The listing builds one solid part. Answer for the finished solid, in the listing's coordinates (mm). Face numbers are marked on the shaded views. A direction names the side the tool comes from. Round coordinates to 2 decimals unless told otherwise and drop trailing zeros. Write each loop counter-clockwise with the first axis right and the second up, starting at its lowest first coordinate (ties: lowest second). Pieces come first, ordered by that corner, then holes. Notation, with made-up numbers: (74, 88.5) - (121, 88.5) arc R21 cw to (121, 104.5) - close; hole circle Ø8 at (-28, 38.25). An arc over 180 degrees is marked (long way). Return JSON: item names as keys, results as strings. Group by question number.
(1) Determine the mould class of the marked faces 3, 4 and 5 for opening direction Y: +Y half, -Y half, draft (parallel to the pull), parting line (faces both ways), or undercut.
(2) Each of these flat-tipped pins is pushed along its axis until it touches: pin 1 (0.9 mm diameter, centred on y = -1.5, z = 3, fed in from -X); pin 2 (10.5 mm diameter, centred on x = 3.5, y = -6, fed in from +Z); pin 3 (1.8 mm diameter, centred on y = 4.5, z = 5, fed in from -X); pin 4 (5 mm diameter, centred on y = -28, z = 4, fed in from +X). Where does it stop, or does it pass through?
(3) Section A-A, the plane x = 0 is taken. Write down the section's boundary in (y, z).
(4) Section C-C, the plane x = -9 is taken. Write down the section's boundary in (y, z).
(5) Find the intervals of material crossed by line 1 along Y through (x, z) = (0, -1.1); line 2 along Z through (x, y) = (3, -23); line 3 along X through (y, z) = (-6.5, 2), in increasing order. Write a range as [from, to].
(6) Section B-B, the plane y = 16.5 is taken. Write down the section's boundary in (x, z), then the cut area to 3 significant figures.
(7) Section D-D, the plane y = -27 is taken. Write down the section's boundary in (x, z).
(8) Which of the six approach directions +Z, -Z, +X, -X, +Y, -Y give full straight-line access (tool end or side, diameter ignored) to the marked faces 1 and 2?
```python
from build123d import *

# Parameters (mm, degrees)
F1_DEPTH  = 6.35
F0_R      = 4.7625
F2_DEPTH  = 2.794
F4_DEPTH  = 1.5875
F6_DEPTH  = 6.35
F8_W      = 1.87325
F8_H      = 21.43125
F9_DEPTH  = 2.794
F11_DEPTH = 0.889
F12_R     = 1.27
F13_R     = 1.27


with BuildPart() as f1:
    # F0 (on Top) → F1 (new body)
    with BuildSketch(Plane.XY):
        with BuildLine():
            ThreePointArc((13.890625, 10.715625), (0, 24.60625), (-13.890625, 10.715625))
            Line((-13.890625, 10.715625), (-13.890625, -10.715625))
            ThreePointArc((-13.890625, -10.715625), (0, -24.60625), (13.890625, -10.715625))
            Line((13.890625, -10.715625), (13.890625, 10.715625))
        make_face()
    extrude(amount=F1_DEPTH)

    # F0 (on Top) → F2 (join)
    with BuildSketch(Plane.XY):
        with BuildLine():
            ThreePointArc((17.065625, 24.60625), (0, 41.671875), (-17.065625, 24.60625))
            Line((-17.065625, 24.60625), (-17.065625, -24.60625))
            ThreePointArc((-17.065625, -24.60625), (0, -41.671875), (17.065625, -24.60625))
            Line((17.065625, -24.60625), (17.065625, 24.60625))
        make_face()
        with Locations((0, -33.734375)):
            Circle(F0_R, mode=Mode.SUBTRACT)
        with BuildLine():
            ThreePointArc((-14.684375, 10.715625), (0, 25.4), (14.684375, 10.715625))
            Line((14.684375, 10.715625), (14.684375, -10.715625))
            ThreePointArc((14.684375, -10.715625), (0, -25.4), (-14.684375, -10.715625))
            Line((-14.684375, -10.715625), (-14.684375, 10.715625))
        make_face(mode=Mode.SUBTRACT)
        with Locations((0, 33.734375)):
            Circle(F0_R, mode=Mode.SUBTRACT)
        with BuildLine():
            Line((14.684375, -10.715625), (14.684375, 10.715625))
            ThreePointArc((14.684375, 10.715625), (0, 25.4), (-14.684375, 10.715625))
            Line((-14.684375, 10.715625), (-14.684375, -10.715625))
            ThreePointArc((-14.684375, -10.715625), (0, -25.4), (14.684375, -10.715625))
        make_face()
        with BuildLine():
            Line((-13.890625, -10.715625), (-13.890625, 10.715625))
            ThreePointArc((-13.890625, 10.715625), (0, 24.60625), (13.890625, 10.715625))
            Line((13.890625, 10.715625), (13.890625, -10.715625))
            ThreePointArc((13.890625, -10.715625), (0, -24.60625), (-13.890625, -10.715625))
        make_face(mode=Mode.SUBTRACT)
        with BuildLine():
            ThreePointArc((13.890625, 10.715625), (0, 24.60625), (-13.890625, 10.715625))
            Line((-13.890625, 10.715625), (-13.890625, -10.715625))
            ThreePointArc((-13.890625, -10.715625), (0, -24.60625), (13.890625, -10.715625))
            Line((13.890625, -10.715625), (13.890625, 10.715625))
        make_face()
    extrude(amount=-F2_DEPTH)

    # F3 (on face) → F4 (join)
    with BuildSketch(Plane(origin=(0, 0, -2.794), x_dir=(1, 0, 0), z_dir=(0, 0, -1))):
        with BuildLine():
            ThreePointArc((17.065625, 24.60625), (0, 41.671875), (-17.065625, 24.60625))
            Line((-17.065625, 24.60625), (-17.065625, -24.60625))
            ThreePointArc((-17.065625, -24.60625), (0, -41.671875), (17.065625, -24.60625))
            Line((17.065625, -24.60625), (17.065625, 24.60625))
        make_face()
    extrude(amount=F4_DEPTH)

    # F5 (on face) → F6 (cut, through all)
    with BuildSketch(Plane.XY.offset(6.35)):
        with BuildLine():
            ThreePointArc((10.715625, 10.715625), (0, 21.43125), (-10.715625, 10.715625))
            Line((-10.715625, 10.715625), (-10.715625, -10.715625))
            ThreePointArc((-10.715625, -10.715625), (0, -21.43125), (10.715625, -10.715625))
            Line((10.715625, -10.715625), (10.715625, 10.715625))
        make_face()
    extrude(amount=-F6_DEPTH, mode=Mode.SUBTRACT)

    # F8 (on face) → F9 (cut, through all)
    with BuildSketch(Plane.XY):
        with Locations((16.129, 0)):
            Rectangle(F8_W, F8_H)
        with Locations((-16.129, 0)):
            Rectangle(F8_W, F8_H)
    extrude(amount=-F9_DEPTH, mode=Mode.SUBTRACT)

    # F10 (on mid) → F11 (cut, symmetric)
    with BuildSketch(Plane.XY.offset(3.175)):
        with BuildLine():
            Line((14.684375, -10.715625), (14.684375, 10.715625))
            ThreePointArc((14.684375, 10.715625), (0, 25.4), (-14.684375, 10.715625))
            Line((-14.684375, 10.715625), (-14.684375, -10.715625))
            ThreePointArc((-14.684375, -10.715625), (0, -25.4), (14.684375, -10.715625))
        make_face()
        with BuildLine():
            ThreePointArc((-12.5042083333, 10.715625), (0, 23.2198333333), (12.5042083333, 10.715625))
            Line((12.5042083333, 10.715625), (12.5042083333, -10.715625))
            ThreePointArc((12.5042083333, -10.715625), (0, -23.2198333333), (-12.5042083333, -10.715625))
            Line((-12.5042083333, -10.715625), (-12.5042083333, 10.715625))
        make_face(mode=Mode.SUBTRACT)
    extrude(amount=F11_DEPTH, both=True, mode=Mode.SUBTRACT)

    # F12
    f12_edges = [f1.edges().sort_by_distance(p)[0] for p in [
        (15.192375, -10.715625, -1.397),
        (15.192375, 10.715625, -1.397),
        (-15.192375, 10.715625, -1.397),
        (-15.192375, -10.715625, -1.397),
    ]]
    fillet(f12_edges, radius=F12_R)

    # F13
    f13_edges = [f1.edges().sort_by_distance(p)[0] for p in [
        (16.764, -10.715625, 0),
        (16.764, 10.715625, 0),
        (16.764, -10.715625, -2.794),
        (16.764, 10.715625, -2.794),
        (-16.764, -10.715625, 0),
        (-16.764, -10.715625, -2.794),
        (-16.764, 10.715625, 0),
        (-16.764, 10.715625, -2.794),
    ]]
    fillet(f13_edges, radius=F13_R)


solid = f1.part
```
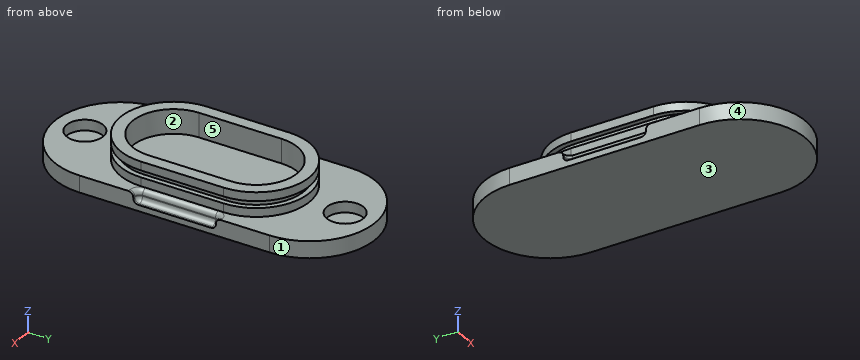
Working result:
{
 "1": {"face 3": "draft", "face 4": "-Y half", "face 5": "undercut"},
 "2": {"pin 1": "stops at x = -12.5", "pin 2": "stops at z = 0", "pin 3": "stops at x = -13.89", "pin 4": "passes through"},
 "3": {"outline": "(-41.67, -4.38) - (41.67, -4.38) - (41.67, 0) - (38.5, 0) - (38.5, -2.79) - (28.97, -2.79) - (28.97, 0) - (24.61, 0) - (24.61, 2.29) - (23.22, 2.29) - (23.22, 4.06) - (24.61, 4.06) - (24.61, 6.35) - (21.43, 6.35) - (21.43, 0) - (-21.43, 0) - (-21.43, 6.35) - (-24.61, 6.35) - (-24.61, 4.06) - (-23.22, 4.06) - (-23.22, 2.29) - (-24.61, 2.29) - (-24.61, 0) - (-28.97, 0) - (-28.97, -2.79) - (-38.5, -2.79) - (-38.5, 0) - (-41.67, 0) - close"},
 "4": {"outline": "(-39.11, -4.38) - (39.11, -4.38) - (39.11, 0) - (21.3, 0) - (21.3, 2.29) - (19.4, 2.29) - (19.4, 4.06) - (21.3, 4.06) - (21.3, 6.35) - (16.53, 6.35) - (16.53, 0) - (-16.53, 0) - (-16.53, 6.35) - (-21.3, 6.35) - (-21.3, 4.06) - (-19.4, 4.06) - (-19.4, 2.29) - (-21.3, 2.29) - (-21.3, 0) - (-39.11, 0) - close"},
 "5": {"line 1": "y = [-41.67, -38.5], [-28.97, 28.97], [38.5, 41.67]", "line 2": "z = [-4.38, 2.29], [4.06, 6.35]", "line 3": "x = [-13.89, -10.72], [10.72, 13.89]"},
 "6": {"outline": "(-17.07, -4.38) - (17.07, -4.38) - (17.07, 0) - (12.63, 0) - (12.63, 2.29) - (11.09, 2.29) - (11.09, 4.06) - (12.63, 4.06) - (12.63, 6.35) - (9.02, 6.35) - (9.02, 0) - (-9.02, 0) - (-9.02, 6.35) - (-12.63, 6.35) - (-12.63, 4.06) - (-11.09, 4.06) - (-11.09, 2.29) - (-12.63, 2.29) - (-12.63, 0) - (-17.07, 0) - close", "area": "190 mm^2"},
 "7": {"outline": "(-16.9, -4.38) - (16.9, -4.38) - (16.9, 0) - (-16.9, 0) - close"},
 "8": {"face 1": "+Z, -Z, +Y", "face 2": "+Z"}
}
